Autodesk Inventor part; units mm, degrees
ref_plane "YZ Plane" through (0, 0, 0) normal (1, 0, 0) x (0, 1, 0)
ref_plane "XZ Plane" through (0, 0, 0) normal (0, 1, 0) x (-1, 0, 0)
ref_plane "XY Plane" through (0, 0, 0) normal (0, 0, 1) x (1, 0, 0)
sketch "Sketch1" plane through (0, 0, 0) normal (0, 0, 1) x (1, 0, 0)
  line L0 (0, 0) -> (-12.7, 0) construction
  line L1 (-12.7, 0) -> (-12.7, 53.975) construction
  line L2 (-12.7, 53.975) -> (0, 53.975) construction
  line L3 (0, 53.975) -> (0, 0) construction
  line L4 (-12.7, 53.975) -> (-25.4, 53.975) construction
  line L5 (-12.7, 53.975) -> (0, 53.975) construction
  line L6 (-25.4, 53.975) -> (-25.4, 0) construction
  line L7 (-25.4, 0) -> (-12.7, 0) construction
  circle A0 centre (-12.7, 6.35) radius 6.35 construction
  circle A1 centre (-12.7, 47.625) radius 6.35 construction
  line L8 (-12.7, 47.625) -> (-18.1993, 50.8) construction
  line L9 (-12.7, 47.625) -> (-6.35, 47.625) construction
  line L10 (-12.7, 47.625) -> (-7.2007, 50.8) construction
  line L11 (-12.7, 47.625) -> (-6.35, 47.625) construction
  line L12 (0, 0) -> (-25.4, 0)
  line L13 (0, 0) -> (0, -1.5875)
  line L14 (0, 0) -> (1.5875, 0) construction
  line L15 (0, -1.5875) -> (-26.9875, -1.5875)
  arc A2 (-7.2007, 50.8) -> (-18.1993, 50.8) centre (-12.7, 47.625) ccw
  line L16 (-7.2007, 50.8) -> (0, 38.328)
  line L17 (-7.2007, 50.8) -> (7.2007, 50.8) construction
  line L18 (-18.1993, 50.8) -> (-24.5493, 39.8015)
  line L19 (-18.1993, 50.8) -> (-5.4993, 50.8) construction
  line L20 (-25.4, 0) -> (-25.4, 36.6265)
  line L21 (-19.5741, 51.5937) -> (-26.1368, 40.2268)
  line L22 (-26.9875, -1.5875) -> (-26.9875, 37.0518)
  arc A3 (-26.1368, 40.2268) -> (-26.9875, 37.0518) centre (-20.6375, 37.0518) ccw
  arc A4 (-24.5493, 39.8015) -> (-25.4, 36.6265) centre (-19.05, 36.6265) ccw
  line L23 (-5.8259, 51.5937) -> (1.3748, 39.1217)
  arc A5 (-5.8259, 51.5937) -> (-19.5741, 51.5937) centre (-12.7, 47.625) ccw
  arc A6 (0, 38.328) -> (1.3748, 39.1217) centre (0.6874, 38.7248) ccw
  point P0 (-25.4, 38.328)
  dimension "d0" = 12.7
  dimension "d1" = 53.975
  dimension "d2" = 12.7
  dimension "d3" = 180
  dimension "d4" = 53.975
  dimension "d5" = 90
  dimension "d6" = 12.7
  dimension "d7" = 12.7
  dimension "d8" = 6.35
  dimension "d9" = 6.35
  dimension "d10" = 6.35
  dimension "d11" = 150
  dimension "d12" = 6.35
  dimension "d13" = 30
  dimension "d14" = 1.5875
  dimension "d15" = 90
  dimension "d16" = 26.9875
  dimension "d17" = 6.35
  dimension "d18" = 60
  dimension "d19" = 120
  dimension "d20" = 90
  dimension "d21" = 1.5875
  dimension "d22" = 6.35
  dimension "d23" = 6.35
  dimension "d24" = 1.5875
  dimension "d25" = 7.9375
  dimension "d26" = 0
extrude "Extrusion1" add sketch "Sketch1" along normal blind 1689.1
sketch "Sketch2" plane through (-26.9875, -1.5875, 0) normal (-1, 0, 0) x (0, 0, 1)
  line L0 (0, 38.6393) -> (0, 0)
  line L1 (0, 0) -> (1689.1, 0)
  line L2 (1689.1, 38.6393) -> (1689.1, 0)
  line L3 (0, 38.6393) -> (1689.1, 38.6393)
  point P0 (0, 1.5875)
  point P1 (1651, 19.05)
  dimension "d29" = 19.05
  dimension "d30" = 38.1
hole "Hole1" at (-26.9875, 17.4625, 1651) direction (1, 0, 0) diameter 9.525 end through all
sketch "Sketch3" plane through (-26.9875, -1.5875, 0) normal (-1, 0, 0) x (0, 0, 1)
  circle A0 centre (1651, 19.05) radius 4.7625
  line L0 (0, 38.6393) -> (0, 0)
  line L1 (0, 0) -> (1689.1, 0)
  line L2 (1689.1, 38.6393) -> (1689.1, 0)
  line L3 (0, 38.6393) -> (1689.1, 38.6393)
  circle A1 centre (31.75, 19.05) radius 4.7625
  line L4 (15.875, 28.575) -> (15.875, 25.4) construction
  line L5 (15.875, 28.575) -> (15.875, 31.75) construction
  line L6 (12.7, 28.575) -> (12.7, 31.75) construction
  line L7 (12.7, 28.575) -> (12.7, 25.4) construction
  line L8 (15.875, 12.7) -> (15.875, 15.875) construction
  line L9 (12.7, 12.7) -> (12.7, 15.875) construction
  line L10 (15.875, 12.7) -> (15.875, 9.525) construction
  line L11 (12.7, 12.7) -> (12.7, 9.525) construction
  arc A2 (15.875, 25.4) -> (15.875, 31.75) centre (15.875, 28.575) ccw
  arc A3 (12.7, 31.75) -> (12.7, 25.4) centre (12.7, 28.575) ccw
  arc A4 (15.875, 9.525) -> (15.875, 15.875) centre (15.875, 12.7) ccw
  arc A5 (12.7, 15.875) -> (12.7, 9.525) centre (12.7, 12.7) ccw
  line L12 (15.875, 31.75) -> (12.7, 31.75)
  line L13 (15.875, 25.4) -> (12.7, 25.4)
  line L14 (15.875, 15.875) -> (12.7, 15.875)
  line L15 (15.875, 9.525) -> (12.7, 9.525)
  point P0 (0, 1.5875)
  dimension "d45" = 12.7
  dimension "d46" = 15.875
  dimension "d47" = 31.75
  dimension "d48" = 12.7
  dimension "d49" = 15.875
  dimension "d50" = 9.525
  dimension "d51" = 19.05
  dimension "d52" = 12.7
  dimension "d53" = 12.7
  dimension "d54" = 28.575
  dimension "d55" = 28.575
  dimension "d56" = 3.175
  dimension "d57" = 3.175
  dimension "d58" = 3.175
  dimension "d59" = 3.175
  dimension "d60" = 3.175
  dimension "d61" = 3.175
  dimension "d62" = 3.175
  dimension "d63" = 3.175
  dimension "d64" = 3.175
  dimension "d65" = 3.175
  dimension "d66" = 3.175
  dimension "d67" = 3.175
extrude "Extrusion2" cut sketch "Sketch3" against normal blind 25.4 contours A1 | L13 A3 L12 A2 | L15 A5 L14 A4
sketch "Sketch4" plane through (-26.9875, -1.5875, 0) normal (-1, 0, 0) x (0, 0, 1)
  line L0 (12.7, 15.875) -> (15.875, 15.875)
  arc A0 (15.875, 9.525) -> (15.875, 15.875) centre (15.875, 12.7) ccw
  line L1 (15.875, 9.525) -> (12.7, 9.525)
  arc A1 (12.7, 15.875) -> (12.7, 9.525) centre (12.7, 12.7) ccw
  line L2 (12.7, 31.75) -> (15.875, 31.75)
  arc A2 (15.875, 25.4) -> (15.875, 31.75) centre (15.875, 28.575) ccw
  line L3 (15.875, 25.4) -> (12.7, 25.4)
  arc A3 (12.7, 31.75) -> (12.7, 25.4) centre (12.7, 28.575) ccw
  circle A4 centre (31.75, 19.05) radius 4.7625
  circle A5 centre (1651, 19.05) radius 4.7625
  line L4 (0, 38.6393) -> (0, 0)
  line L5 (0, 0) -> (1689.1, 0)
  line L6 (1689.1, 38.6393) -> (1689.1, 0)
  line L7 (0, 38.6393) -> (1689.1, 38.6393)
  point P0 (0, 1.5875)
  point P1 (101.6, 25.4)
  point P2 (88.9, 12.7)
  point P3 (76.2, 25.4)
  point P4 (63.5, 12.7)
  dimension "d70" = 63.5
  dimension "d71" = 76.2
  dimension "d72" = 88.9
  dimension "d73" = 101.6
  dimension "d74" = 12.7
  dimension "d77" = 12.7
  dimension "d120" = 25.4
  dimension "d121" = 25.4
hole "Hole2" at (-26.9875, 23.8125, 101.6) at (-26.9875, 11.1125, 88.9) at (-26.9875, 23.8125, 76.2) at (-26.9875, 11.1125, 63.5) direction (1, 0, 0) diameter 6.35 end through all
sketch "Sketch6" plane through (-26.9875, -1.5875, 0) normal (-1, 0, 0) x (0, 0, 1)
  circle A0 centre (76.2, 25.4) radius 3.175
  circle A1 centre (101.6, 25.4) radius 3.175
  circle A2 centre (88.9, 12.7) radius 3.175
  circle A3 centre (63.5, 12.7) radius 3.175
  line L0 (12.7, 15.875) -> (15.875, 15.875)
  arc A4 (15.875, 9.525) -> (15.875, 15.875) centre (15.875, 12.7) ccw
  line L1 (15.875, 9.525) -> (12.7, 9.525)
  arc A5 (12.7, 15.875) -> (12.7, 9.525) centre (12.7, 12.7) ccw
  line L2 (12.7, 31.75) -> (15.875, 31.75)
  arc A6 (15.875, 25.4) -> (15.875, 31.75) centre (15.875, 28.575) ccw
  line L3 (15.875, 25.4) -> (12.7, 25.4)
  arc A7 (12.7, 31.75) -> (12.7, 25.4) centre (12.7, 28.575) ccw
  circle A8 centre (31.75, 19.05) radius 4.7625
  circle A9 centre (1651, 19.05) radius 4.7625
  line L4 (0, 38.6393) -> (0, 0)
  line L5 (0, 0) -> (1689.1, 0)
  line L6 (1689.1, 38.6393) -> (1689.1, 0)
  line L7 (0, 38.6393) -> (1689.1, 38.6393)
  line L8 (787.4, 6.35) -> (838.2, 6.35)
  line L9 (838.2, 6.35) -> (838.2, 31.75)
  line L10 (838.2, 31.75) -> (787.4, 31.75)
  line L11 (787.4, 31.75) -> (787.4, 6.35)
  line L12 (901.7, 6.35) -> (952.5, 6.35)
  line L13 (952.5, 6.35) -> (952.5, 31.75)
  line L14 (952.5, 31.75) -> (901.7, 31.75)
  line L15 (901.7, 31.75) -> (901.7, 6.35)
  point P0 (0, 1.5875)
  dimension "d98" = 50.8
  dimension "d99" = 25.4
  dimension "d100" = 50.8
  dimension "d101" = 25.4
  dimension "d102" = 787.4
  dimension "d103" = 901.7
  dimension "d104" = 6.35
  dimension "d105" = 6.35
extrude "Extrusion3" cut sketch "Sketch6" against normal blind 25.4 contours L11 L10 L9 L8 | L15 L14 L13 L12
sketch "Sketch8" plane through (-26.9875, -1.5875, 0) normal (-1, 0, 0) x (0, 0, 1)
  line L0 (838.2, 31.75) -> (838.2, 6.35)
  line L1 (838.2, 6.35) -> (787.4, 6.35)
  line L2 (787.4, 6.35) -> (787.4, 31.75)
  line L3 (787.4, 31.75) -> (838.2, 31.75)
  line L4 (952.5, 31.75) -> (952.5, 6.35)
  line L5 (952.5, 6.35) -> (901.7, 6.35)
  line L6 (901.7, 6.35) -> (901.7, 31.75)
  line L7 (901.7, 31.75) -> (952.5, 31.75)
  circle A0 centre (76.2, 25.4) radius 3.175
  circle A1 centre (101.6, 25.4) radius 3.175
  circle A2 centre (88.9, 12.7) radius 3.175
  circle A3 centre (63.5, 12.7) radius 3.175
  line L8 (12.7, 15.875) -> (15.875, 15.875)
  arc A4 (15.875, 9.525) -> (15.875, 15.875) centre (15.875, 12.7) ccw
  line L9 (15.875, 9.525) -> (12.7, 9.525)
  arc A5 (12.7, 15.875) -> (12.7, 9.525) centre (12.7, 12.7) ccw
  line L10 (12.7, 31.75) -> (15.875, 31.75)
  arc A6 (15.875, 25.4) -> (15.875, 31.75) centre (15.875, 28.575) ccw
  line L11 (15.875, 25.4) -> (12.7, 25.4)
  arc A7 (12.7, 31.75) -> (12.7, 25.4) centre (12.7, 28.575) ccw
  circle A8 centre (31.75, 19.05) radius 4.7625
  circle A9 centre (1651, 19.05) radius 4.7625
  line L12 (0, 38.6393) -> (0, 0)
  line L13 (0, 0) -> (1689.1, 0)
  line L14 (1689.1, 38.6393) -> (1689.1, 0)
  line L15 (0, 38.6393) -> (1689.1, 38.6393)
  point P0 (0, 1.5875)
  point P1 (965.2, 19.05)
  point P2 (774.7, 19.05)
  dimension "d122" = 19.05
  dimension "d123" = 19.05
  dimension "d124" = 190.5
  dimension "d125" = 774.7
hole "Hole5" at (-26.9875, 17.4625, 965.2) at (-26.9875, 17.4625, 774.7) direction (1, 0, 0) diameter 6.35 end through all
sketch "Sketch9" plane through (0, -1.5875, 0) normal (0, -1, 0) x (1, 0, 0)
  line L0 (-26.9875, 0) -> (0, 0)
  line L1 (0, 0) -> (0, 1689.1)
  line L2 (-26.9875, 1689.1) -> (0, 1689.1)
  point P0 (-12.7, 25.4)
  point P1 (-12.7, 1676.4)
  dimension "d135" = 12.7
  dimension "d136" = 12.7
  dimension "d137" = 12.7
  dimension "d138" = 25.4
hole "Hole6" at (-12.7, -1.5875, 25.4) at (-12.7, -1.5875, 1676.4) direction (0, 1, 0) diameter 6.35 depth 25.4 tip angle 118
sketch "Sketch10" plane through (0, 0, 1689.1) normal (0, 0, 1) x (1, 0, 0)
  line L0 (0, 0) -> (-25.4, 0)
  line L1 (-25.4, 0) -> (-25.4, 36.6265)
  arc A0 (-24.5493, 39.8015) -> (-25.4, 36.6265) centre (-19.05, 36.6265) ccw
  line L2 (-24.5493, 39.8015) -> (-18.1993, 50.8)
  arc A1 (-7.2007, 50.8) -> (-18.1993, 50.8) centre (-12.7, 47.625) ccw
  line L3 (-7.2007, 50.8) -> (0, 38.328)
  arc A2 (0, 38.328) -> (1.3748, 39.1217) centre (0.6874, 38.7248) ccw
  line L4 (1.3748, 39.1217) -> (-5.8259, 51.5937)
  arc A3 (-5.8259, 51.5937) -> (-19.5741, 51.5937) centre (-12.7, 47.625) ccw
  line L5 (-19.5741, 51.5937) -> (-26.1368, 40.2268)
  arc A4 (-26.1368, 40.2268) -> (-26.9875, 37.0518) centre (-20.6375, 37.0518) ccw
  line L6 (-26.9875, 37.0518) -> (-26.9875, -1.5875)
  line L7 (-26.9875, -1.5875) -> (0, -1.5875)
  line L8 (0, -1.5875) -> (0, 0)
extrude "Extrusion4" cut sketch "Sketch10" against normal blind 19.05
sketch "Sketch11" plane through (-26.9875, -1.5875, 0) normal (-1, 0, 0) x (0, 0, 1)
  line L0 (1670.05, 0) -> (1670.05, 38.6393)
  line L1 (0, 38.6393) -> (1670.05, 38.6393)
  line L2 (0, 38.6393) -> (0, 0)
  line L3 (0, 0) -> (1670.05, 0)
  circle A0 centre (965.2, 19.05) radius 3.175
  circle A1 centre (774.7, 19.05) radius 3.175
  line L4 (838.2, 31.75) -> (838.2, 6.35)
  line L5 (838.2, 6.35) -> (787.4, 6.35)
  line L6 (787.4, 6.35) -> (787.4, 31.75)
  line L7 (787.4, 31.75) -> (838.2, 31.75)
  line L8 (952.5, 31.75) -> (952.5, 6.35)
  line L9 (952.5, 6.35) -> (901.7, 6.35)
  line L10 (901.7, 6.35) -> (901.7, 31.75)
  line L11 (901.7, 31.75) -> (952.5, 31.75)
  circle A2 centre (76.2, 25.4) radius 3.175
  circle A3 centre (101.6, 25.4) radius 3.175
  circle A4 centre (88.9, 12.7) radius 3.175
  circle A5 centre (63.5, 12.7) radius 3.175
  line L12 (12.7, 15.875) -> (15.875, 15.875)
  arc A6 (15.875, 9.525) -> (15.875, 15.875) centre (15.875, 12.7) ccw
  line L13 (15.875, 9.525) -> (12.7, 9.525)
  arc A7 (12.7, 15.875) -> (12.7, 9.525) centre (12.7, 12.7) ccw
  line L14 (12.7, 31.75) -> (15.875, 31.75)
  arc A8 (15.875, 25.4) -> (15.875, 31.75) centre (15.875, 28.575) ccw
  line L15 (15.875, 25.4) -> (12.7, 25.4)
  arc A9 (12.7, 31.75) -> (12.7, 25.4) centre (12.7, 28.575) ccw
  circle A10 centre (31.75, 19.05) radius 4.7625
  circle A11 centre (1651, 19.05) radius 4.7625
  point P0 (0, 1.5875)
  point P1 (1600.2, 18.7956)
  dimension "d148" = 19.8438
  dimension "d149" = 69.85
hole "Hole7" at (-26.9875, 17.2081, 1600.2) direction (1, 0, 0) diameter 6.35 end through all
properties part number "2in rail right" material "Steel, Alloy"
Input: part model. Units: mm. Frame: model coordinates. A direction names the side the tool comes from. Give positions to 0.01 mm unless a question says otherwise; leave off trailing zeros. Order: outer loops, then holes, each group sorted by start corner. A loop starts at its lowest first (then second) coordinate and runs counter-clockwise, first axis right, second up. Notation, with made-up numbers: (18.25, 8) -> (61.25, 8) arc R14 cw to (61.25, 22) -> close; hole circle Ø11 at (68, 61). An arc over 180 degrees is marked (long way). Use one line per item in the form item = value.
1) Section A-A, the plane z = 563. Return loops of the section in (x, y) (1 decimal).
Response values:
outline = (-27, -1.6) -> (0, -1.6) -> (0, 0) -> (-25.4, 0) -> (-25.4, 36.6) arc R6.3 cw to (-24.5, 39.8) -> (-18.2, 50.8) arc R6.4 cw to (-7.2, 50.8) -> (0, 38.3) arc R0.8 ccw to (1.4, 39.1) -> (-5.8, 51.6) arc R7.9 ccw to (-19.6, 51.6) -> (-26.1, 40.2) arc R6.3 ccw to (-27, 37.1) -> close
2) First-contact query: pin 1 Ø0.5 at (x, z) = (-26.5, 917) entering from +Y; pin 2 Ø6 at (y, z) = (28, 417.5) entering from +X; pin 3 Ø7.5 at (x, z) = (-19, 909) entering from +Y. Flat tips, straight axial feed; report the tip coordinate or a pass-through.
Response values:
pin_1 = 40.02
pin_2 = -25.4
pin_3 = 55.14
3) Mould query, pull axis Z, two halves, no side actions, for faces 3 (the flat face through (-13, -1.588, 823)), 4 (the flat face through (-26.5, 22.9, 0)), 5 (the flat face through (-26.5, 22.9, 1670.05)). Classes: pulls with the +Z half, pulls with the -Z half, needs draft (parallel to the pull), parting line crosses it, or undercut.
Response values:
face_3 = needs draft
face_4 = pulls with the -Z half
face_5 = pulls with the +Z half
4) Line query: probe 1 along Y at (x, z) = (-26.5, 1651) (1 decimal); probe 2 along Y at (x, z) = (-26.3, 1600.2); probe 3 along X at (y, z) = (5.5, 1356). Output: solid intervals per line, ascending.
Response values:
probe_1 = -1.6 to 12.7, 22.2 to 39.5
probe_2 = -1.59 to 14.03, 20.38 to 39.93
probe_3 = -26.99 to -25.4
5) Reachability of faces 1 (the flat face through (-26.988, 4.6, 823.3)), 2 (the flat face through (-25.4, 34, 823)) from +Z, -Z, +X, -X, +Y, -Y: full face, straight path, thin tool, end or side. Return the list, or none.
Response values:
face_1 = +Z, -Z, -X, +Y, -Y
face_2 = +Z, -Z, +X
